Autodesk Inventor part; units mm, degrees
ref_plane "YZ Plane" through (0, 0, 0) normal (1, 0, 0) x (0, 1, 0)
ref_plane "XZ Plane" through (0, 0, 0) normal (0, 1, 0) x (-1, 0, 0)
ref_plane "XY Plane" through (0, 0, 0) normal (0, 0, 1) x (1, 0, 0)
sketch "Skizze2" plane through (0, 0, 0) normal (1, 0, 0) x (0, 1, 0)
  line L0 (47.4748, 12) -> (11.7576, 25)
  line L1 (0, 0) -> (48.6481, 0)
  line L2 (47.4748, 12) -> (47.4748, 20.6434)
  line L3 (47.4748, 20.6434) -> (31.9696, 20.6434)
  line L4 (6.2626, 30) -> (31.9696, 20.6434)
  line L5 (4, 30) -> (4, 26.75)
  line L6 (4, 26.75) -> (0, 26.75)
  line L7 (6.2626, 30) -> (4, 30)
  line L8 (11.7576, 25) -> (0, 25)
  line L9 (0, 25) -> (0, 26.75)
  line L10 (0, 0) -> (0, 25) construction
  dimension "d21" = 24
  dimension "d22" = 20
  dimension "d115" = 15.5052
  dimension "d164" = 60
  dimension "d166" = 53.5
  dimension "d167" = 50
  dimension "d168" = 4
  dimension "d169" = 3.25
  dimension "d170" = 8.6434
  dimension "d171" = 47.4748
revolve "Umdrehung1" add sketch "Skizze2" angle 360 about axis through (0, 0, 0) along (0, 1, 0)
sketch "Skizze15" plane through (0, 47.4748, 0) normal (0, 1, 0) x (1, 0, 0)
  circle A0 centre (0, 0) radius 20.6434
  circle A1 centre (0, 0) radius 12
  line L0 (-5, 18.6434) -> (-5, 22.6434)
  line L1 (-5, 22.6434) -> (5, 22.6434)
  line L2 (5, 22.6434) -> (5, 18.6434)
  line L3 (5, 18.6434) -> (-5, 18.6434)
  line L4 (-5, 18.6434) -> (5, 22.6434) construction
  line L5 (-5, 22.6434) -> (5, 18.6434) construction
  line L6 (-17.1098, -15.6518) -> (-22.1098, -6.9916)
  line L7 (-22.1098, -6.9916) -> (-18.6457, -4.9916)
  line L8 (-18.6457, -4.9916) -> (-13.6457, -13.6518)
  line L9 (-13.6457, -13.6518) -> (-17.1098, -15.6518)
  line L10 (22.1098, -6.9916) -> (17.1098, -15.6518)
  line L11 (17.1098, -15.6518) -> (13.6457, -13.6518)
  line L12 (13.6457, -13.6518) -> (18.6457, -4.9916)
  line L13 (18.6457, -4.9916) -> (22.1098, -6.9916)
  point P0 (0, 20.6434)
  dimension "d129" = 10
  dimension "d130" = 4
  dimension "d131" = 18.6434
  dimension "d134" = 360
extrude "Extrusion12" add sketch "Skizze15" against normal blind 25 contours L2 L3 L0 A0 | A0 L0 L1 L2 | L13 L10 L11 A0 | A0 L11 L12 L13 | L7 L8 L9 A0 | A0 L9 L6 L7
delete faces "Fläche löschen5" heal yes whole lump no faces at (0, 24.7239, -18.6434) (0.5603, 22.4748, -19.4397)
delete faces "Fläche löschen6" heal yes whole lump no faces at (17.1154, 22.4748, 9.2346) (16.1457, 24.7239, 9.3217)
delete faces "Fläche löschen7" heal yes whole lump no faces at (-16.5551, 22.4748, 10.2051) (-16.1457, 24.7239, 9.3217)
ref_plane "Arbeitsebene2" through (-5, 43.4748, -22.6434) normal (0, 1, 0) x (1, 0, 0)
sketch "Skizze16" plane through (-5, 43.4748, -22.6434) normal (0, 1, 0) x (1, 0, 0)
  line L0 (-17.1098, -29.635) -> (-12.1098, -38.2953)
  line L1 (0, 0) -> (10, 0)
  line L2 (2.15, 5.7) -> (7.85, 5.7)
  line L3 (7.85, 5.7) -> (7.85, -5.7)
  line L4 (7.85, -5.7) -> (2.15, -5.7)
  line L5 (2.15, -5.7) -> (2.15, 5.7)
  line L6 (2.15, 5.7) -> (7.85, -5.7) construction
  line L7 (7.85, 5.7) -> (2.15, -5.7) construction
  line L8 (-20.9711, -34.347) -> (-11.0984, -28.647)
  line L9 (-18.1211, -39.2833) -> (-20.9711, -34.347)
  line L10 (-8.2484, -33.5833) -> (-18.1211, -39.2833)
  line L11 (-11.0984, -28.647) -> (-8.2484, -33.5833)
  line L12 (28.1211, -39.2833) -> (18.2484, -33.5833)
  line L13 (30.9711, -34.347) -> (28.1211, -39.2833)
  line L14 (21.0984, -28.647) -> (30.9711, -34.347)
  line L15 (18.2484, -33.5833) -> (21.0984, -28.647)
  point P0 (5, -22.6434)
  point P1 (5, 0)
  dimension "d139" = 5.7
  dimension "d140" = 11.4
  dimension "d143" = 360
extrude "Extrusion13" cut sketch "Skizze16" against normal blind 2
sketch "Skizze17" plane through (-5, 47.4748, -22.6434) normal (0, 1, 0) x (1, 0, 0)
  line L0 (0, 0) -> (10, 0)
  line L1 (5, -22.6434) -> (5, -2.85) construction
  point P0 (-12.1416, -32.5402)
  point P1 (22.1416, -32.5402)
  dimension "d147" = 2.85
  dimension "d150" = 360
hole "Bohrung3" at (0, 47.4748, -19.7934) at (-17.1416, 47.4748, 9.8967) at (17.1416, 47.4748, 9.8967) direction (0, -1, 0) diameter 3.3 depth 15 tip angle 118
fillet "Rundung1" radius 2 1 edges at (0, 47.4748, -12)
properties part number "endkappen"
Verification items for the finished model (mm, model axes). A direction names the side the tool comes from. Coordinates: 2 decimals unless noted, no trailing zeros. Write each loop counter-clockwise with the first axis right and the second up, starting at its lowest first coordinate (ties: lowest second). Pieces come first, ordered by that corner, then holes. Notation, with made-up numbers: (41.25, 21.5) - (100.25, 21.5) arc R17 ccw to (100.25, 39.5) - close; hole circle Ø11 at (11, -31). An arc over 180 degrees is marked (long way). Answer as a JSON object with one key per item and string values.
(1) Cross-section at C-C on y = 19. Record the cut outline in (x, z).
Report:
{"outline": "circle Ø50.73 at (0, 0); hole circle Ø44.73 at (0, 0)"}
(2) Mould release check, pull along Y, two halves, no side actions. Record for faces 1 (the flat face through (15.751, 42.489, 12.385)), 2 (the flat face through (5, 39, -21)), 3 (the conical face through (16.862, 31.656, 9.835)): pulls with the +Y half, pulls with the -Y half, needs draft (parallel to the pull), parting line crosses it, or undercut.
Report:
{"face 1": "undercut", "face 2": "needs draft", "face 3": "pulls with the +Y half"}
(3) Cross-section at A-A on z = 0. Record the cut outline in (x, y).
Report:
{"outline": "(-30, 4) - (-26.75, 4) - (-26.75, 0) - (-25, 0) - (-25, 11.76) - (-12.98, 44.79) arc R2 ccw to (-14.86, 47.47) - (-20.64, 47.47) - (-20.64, 31.97) - (-30, 6.26) - close; (12.98, 44.79) - (25, 11.76) - (25, 0) - (26.75, 0) - (26.75, 4) - (30, 4) - (30, 6.26) - (20.64, 31.97) - (20.64, 47.47) - (14.86, 47.47) arc R2 ccw to start"}
(4) Tool access check on faces 4 (the flat face through (17, 43.475, 12)), 5 (the cylindrical face through (-0.5, 36.91, -18.22)), 6 (the cylindrical face through (-7.509, 5.796, 23.846)), 7 (the flat face through (0, 42, -16.943)). Record the directions out of +Z, -Z, +X, -X, +Y, -Y that give a thin tool (end or side, any length) a straight path to the whole face; none if there is none.
Report:
{"face 4": "none", "face 5": "+Y", "face 6": "-Y", "face 7": "-Z"}
(5) Cross-section at B-B on y = 38.5. Record the cut outline in (x, z).
Report:
{"outline": "(-22.11, 6.99) - (-19.85, 5.68) arc R20.64 ccw to (-5, -20.03) - (-5, -22.64) - (5, -22.64) - (5, -20.03) arc R20.64 ccw to (19.85, 5.68) - (22.11, 6.99) - (17.11, 15.65) - (14.85, 14.34) arc R20.64 ccw to (-14.85, 14.34) - (-17.11, 15.65) - close; hole circle Ø3.3 at (-17.14, 9.9); hole circle Ø30.53 at (0, 0); hole circle Ø3.3 at (0, -19.79); hole circle Ø3.3 at (17.14, 9.9)"}
(6) Thickness scan on line 1 along X through (y, z) = (29.5, 15); line 2 along Z through (x, y) = (1.5, 36.5); line 3 along Z through (x, y) = (18, 23.5). Record the ranges inside material, lowest first.
Report:
{"line 1": "-17.49 to -15.98, -15.46 to -10.9, 10.9 to 15.46, 15.98 to 17.49", "line 2": "-22.64 to -20.48, -19.11 to -15.92, 15.92 to 20.59", "line 3": "-15.46 to -10.27, 10.27 to 15.46"}
(7) Gauge pin test, flat ends, axial feed: pin 1 Ø2 at (x, y) = (8.5, 34) entering from -Z; pin 2 Ø10 at (x, y) = (7, 37) entering from -Z; pin 3 Ø3 at (x, y) = (-13, 32.5) entering from +Z. Record the tip position at first contact, or that the pin passes through.
Report:
{"pin 1": "z = -19.23", "pin 2": "z = -22.64", "pin 3": "z = 17.14"}
